```python
from build123d import *

# Parameters (mm, degrees)
IZIM1_R                     = 2.25
Y_KSEKLIK_EKSTR_ZYON1_DEPTH = 130
IZIM2_R                     = 1.6
KES_EKSTR_ZYON1_DEPTH       = 20


with BuildPart() as part:
    # Çizim1 → Yükseklik-Ekstrüzyon1 (new body)
    with BuildSketch(Plane.XY):
        with BuildLine():
            Line((-9.727729885, 0), (12.272270115, 0))
            Line((12.272270115, 0), (12.272270115, 4))
            Line((12.272270115, 4), (5.522270115, 4))
            Line((5.522270115, 4), (5.522270115, 7))
            ThreePointArc((5.522270115, 7), (1.272270115, 11.25), (-2.977729885, 7))
            Line((-2.977729885, 7), (-2.977729885, 4))
            Line((-2.977729885, 4), (-9.727729885, 4))
            Line((-9.727729885, 4), (-9.727729885, 0))
        make_face()
        with Locations((1.272270115, 7)):
            Circle(IZIM1_R, mode=Mode.SUBTRACT)
    extrude(amount=Y_KSEKLIK_EKSTR_ZYON1_DEPTH)

    # Çizim2 → Kes-Ekstrüzyon1 (cut)
    with BuildSketch(Plane(origin=(0, 8.085148281, 0), x_dir=(1, 0, 0), z_dir=(0, 1, 0))):
        with Locations(Location((8.772270115, -5, 0), (0, 0, 270))):
            Circle(IZIM2_R)
        with Locations(Location((-6.227729885, -5, 0), (0, 0, 270))):
            Circle(IZIM2_R)
        with Locations(Location((-6.227729885, -15, 0), (0, 0, 270))):
            Circle(IZIM2_R)
        with Locations(Location((8.772270115, -15, 0), (0, 0, 270))):
            Circle(IZIM2_R)
        with Locations(Location((8.772270115, -35, 0), (0, 0, 270))):
            Circle(IZIM2_R)
        with Locations(Location((8.772270115, -45, 0), (0, 0, 270))):
            Circle(IZIM2_R)
        with Locations(Location((-6.227729885, -35, 0), (0, 0, 270))):
            Circle(IZIM2_R)
        with Locations(Location((-6.227729885, -45, 0), (0, 0, 270))):
            Circle(IZIM2_R)
        with Locations(Location((-6.227729885, -25, 0), (0, 0, 270))):
            Circle(IZIM2_R)
        with Locations(Location((8.772270115, -25, 0), (0, 0, 270))):
            Circle(IZIM2_R)
        with Locations(Location((-6.227729885, -55, 0), (0, 0, 270))):
            Circle(IZIM2_R)
        with Locations(Location((8.772270115, -55, 0), (0, 0, 270))):
            Circle(IZIM2_R)
        with Locations(Location((8.772270115, -75, 0), (0, 0, 270))):
            Circle(IZIM2_R)
        with Locations(Location((-6.227729885, -75, 0), (0, 0, 270))):
            Circle(IZIM2_R)
        with Locations(Location((8.772270115, -105, 0), (0, 0, 270))):
            Circle(IZIM2_R)
        with Locations(Location((-6.227729885, -105, 0), (0, 0, 270))):
            Circle(IZIM2_R)
        with Locations(Location((-6.227729885, -85, 0), (0, 0, 270))):
            Circle(IZIM2_R)
        with Locations(Location((-6.227729885, -95, 0), (0, 0, 270))):
            Circle(IZIM2_R)
        with Locations(Location((8.772270115, -85, 0), (0, 0, 270))):
            Circle(IZIM2_R)
        with Locations(Location((8.772270115, -95, 0), (0, 0, 270))):
            Circle(IZIM2_R)
        with Locations(Location((8.772270115, -115, 0), (0, 0, 270))):
            Circle(IZIM2_R)
        with Locations(Location((-6.227729885, -115, 0), (0, 0, 270))):
            Circle(IZIM2_R)
        with Locations(Location((-6.227729885, -125, 0), (0, 0, 270))):
            Circle(IZIM2_R)
        with Locations(Location((8.772270115, -125, 0), (0, 0, 270))):
            Circle(IZIM2_R)
    extrude(amount=-KES_EKSTR_ZYON1_DEPTH, mode=Mode.SUBTRACT)


solid = part.part
```
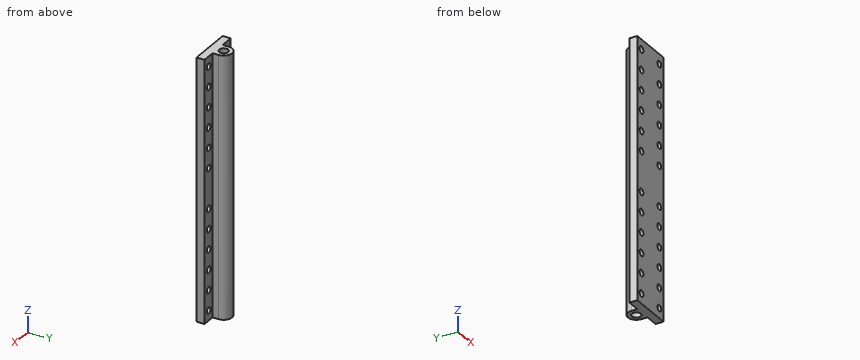
Verification items for the finished model (mm, model axes). Round coordinates to 2 decimals unless told otherwise and drop trailing zeros. Write each loop counter-clockwise with the first axis right and the second up, starting at its lowest first coordinate (ties: lowest second). Pieces come first, ordered by that corner, then holes. Notation, with made-up numbers: (55, 64) - (95, 64) arc R22 ccw to (95, 103) - close; hole circle Ø4 at (-29.75, 7). An arc over 180 degrees is marked (long way). Answer as a JSON object with one key per item and string values. Group by question number.
Q1. Go/stop test with flat-tipped pins: pin 1 Ø5 at (y, z) = (8, 56.5) entering from +X; pin 2 Ø4 at (x, z) = (3.5, 20.5) entering from +Y; pin 3 Ø3.5 at (x, z) = (-6.23, 35) entering from +Y. Record where each tip stops, or that it passes through.
Q2. Section check B-B, the plane y = 1.5. Give the number of separate pieces and of enclosed holes in the cut face, plus the area to 3 significant figures.
Q3. Thickness scan on line 1 (X direction, y = 1.8, z = 15); line 2 (X direction, y = 6.75, z = 19.5); line 3 (Y direction, x = 1.5, z = 31). Record the ranges inside material, lowest first.
Q4. Section check A-A, the plane z = 35. Enter the section's corners in (x, y), plus the area to 3 significant figures.
Found:
{
 "1": {"pin 1": "stops at x = 5.52", "pin 2": "stops at y = 11.24", "pin 3": "stops at y = 4"},
 "2": {"separate pieces": "1", "enclosed holes": "24", "area": "2,670 mm^2"},
 "3": {"line 1": "x = -9.73 to -7.83, -4.63 to 7.17, 10.37 to 12.27", "line 2": "x = -2.98 to -0.96, 3.51 to 5.52", "line 3": "y = 0 to 4.76, 9.24 to 11.24"},
 "4": {"outline": "(-9.73, 0) - (-7.83, 0) - (-7.83, 4) - (-9.73, 4) - close; (-4.63, 0) - (7.17, 0) - (7.17, 4) - (5.52, 4) - (5.52, 7) arc R4.25 ccw to (-2.98, 7) - (-2.98, 4) - (-4.63, 4) - close; (10.37, 0) - (12.27, 0) - (12.27, 4) - (10.37, 4) - close; hole circle Ø4.5 at (1.27, 7)", "area": "100 mm^2"}
}
